Verification items for this drawing (mm, ordinates from the low corner). Give positions to 0.01 mm unless a question says otherwise; leave off trailing zeros. Loops run counter-clockwise (first coordinate to the right, second up) from the corner with the lowest first, then second, coordinate; pieces in that order, holes last. Notation, with made-up numbers: (81, -23) -> (130, -23) arc R21 ccw to (130, 0) -> close; hole circle Ø5 at (21.5, 10.25). An arc over 180 degrees is marked (long way). Answer as a JSON object with one key per item and string values.
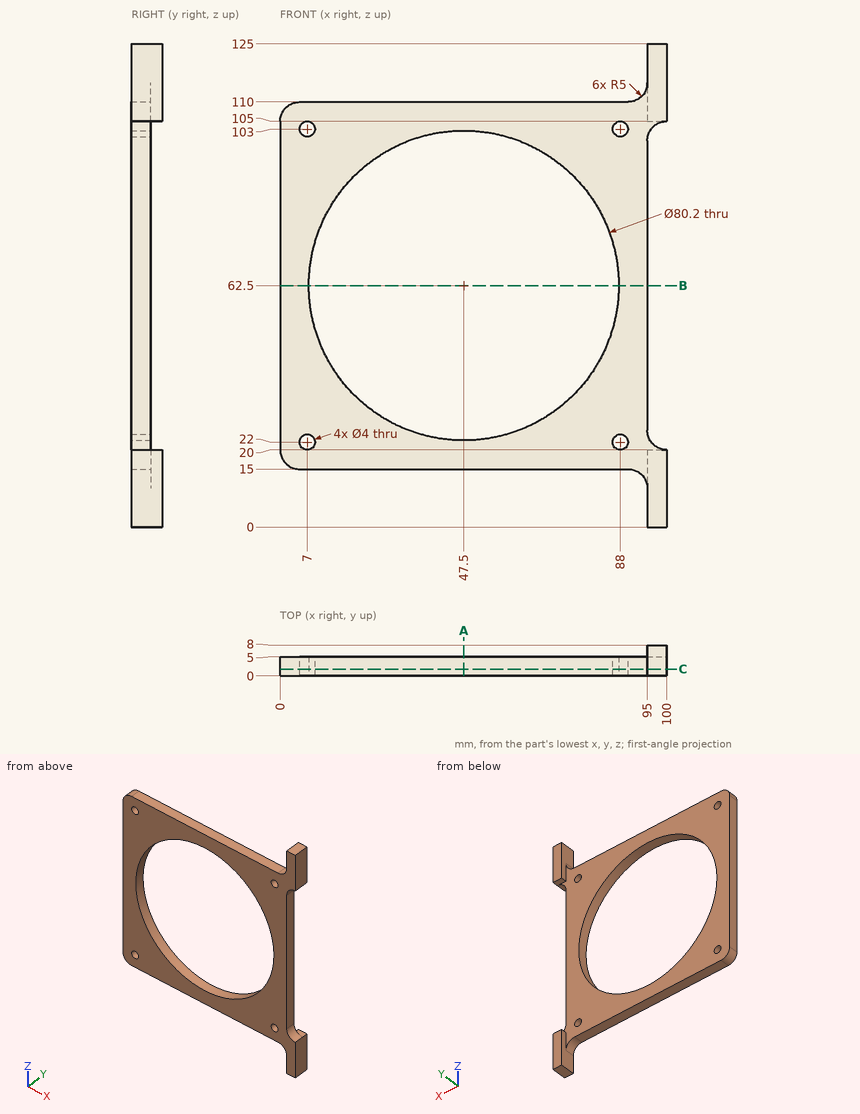
1) Material ranges on line 1 along Z through (x, y) = (88, 3.2); line 2 along X through (y, z) = (3.35, 22); line 3 along Y through (x, z) = (16, 92), recorded low to high. Write a range as from..to.
Geometry check:
{"line 1": "z = 15..20, 24..101, 105..110", "line 2": "x = 0..5, 9..86, 90..96", "line 3": "y = 0..5"}
2) Section check A-A on x = 47.5. Record the cut outline in (y, z).
Geometry check:
{"outline": "(0, 15) -> (5, 15) -> (5, 22.4) -> (0, 22.4) -> close; (0, 102.6) -> (5, 102.6) -> (5, 110) -> (0, 110) -> close"}
3) Section check B-B on z = 62.5. Record the cut outline in (x, y).
Geometry check:
{"outline": "(0, 0) -> (7.4, 0) -> (7.4, 5) -> (0, 5) -> close; (87.6, 0) -> (95, 0) -> (95, 5) -> (87.6, 5) -> close"}
4) Section check C-C on y = 1.75. Count the separate pieces of the cut face and the enclosed holes in it, plus the area to 3 significant figures.
Geometry check:
{"separate pieces": "1", "enclosed holes": "5", "area": "4,130 mm2"}
5) Depth check by flat-ended pin: P1, Ø3, axis at y = 3.5, z = 43.5, coming from the +X side; P2, Ø4, axis at y = 3, z = 119.5, coming from the -X side; P3, Ø4, axis at y = 4.5, z = 13.5, coming from the -X side; P4, Ø2.5, axis at x = 7, z = 103, coming from the -Y side. Enter the tip coordinate at first touch or a pass-through.
Geometry check:
{"P1": "stops at x = 95", "P2": "stops at x = 95", "P3": "stops at x = 2.82", "P4": "passes through"}
